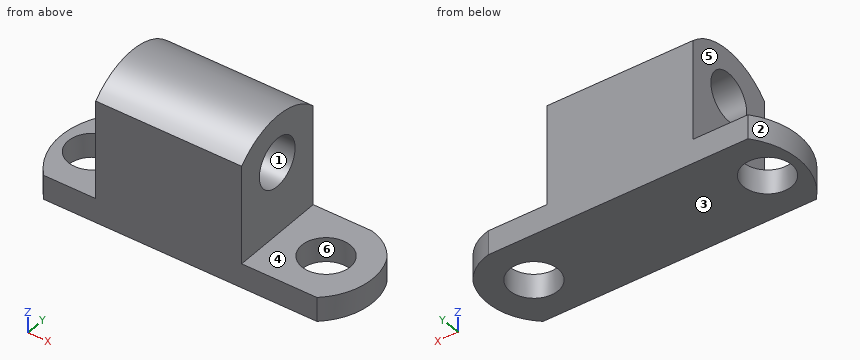
from build123d import *

# Parameters (mm, degrees)
F0_W      = 82.55
F0_H      = 38.1
F1_DEPTH  = 25.4
F2_W      = 25.4
F2_H      = 31.75
F3_DEPTH  = 25.4
F4_W      = 19.05
F4_H      = 31.75
F5_DEPTH  = 25.4
F6_R      = 6.35
F7_DEPTH  = 25.4
F8_R      = 6.35
F9_DEPTH  = 25.4
F11_DEPTH = 38.1
F12_R     = 6.35
F13_DEPTH = 50.8
F15_DEPTH = 50.8
F17_DEPTH = 50.8
F19_DEPTH = 25.4


with BuildPart() as f1:
    # F0 (on Front) → F1 (new body)
    with BuildSketch(Plane.XZ):
        with Locations((41.275, 19.05)):
            Rectangle(F0_W, F0_H)
    extrude(amount=F1_DEPTH)

    # F2 (on face) → F3 (cut)
    with BuildSketch(Plane.XZ.offset(25.4)):
        with Locations((69.85, 22.225)):
            Rectangle(F2_W, F2_H)
    extrude(amount=-F3_DEPTH, mode=Mode.SUBTRACT)

    # F4 (on face) → F5 (cut)
    with BuildSketch(Plane.XZ.offset(25.4)):
        with Locations((9.525, 22.225)):
            Rectangle(F4_W, F4_H)
    extrude(amount=-F5_DEPTH, mode=Mode.SUBTRACT)

    # F6 (on face) → F7 (cut)
    with BuildSketch(Plane.XY.offset(6.35)):
        with Locations((69.85, -12.7)):
            Circle(F6_R)
    extrude(amount=-F7_DEPTH, mode=Mode.SUBTRACT)

    # F8 (on face) → F9 (cut)
    with BuildSketch(Plane.XY.offset(6.35)):
        with Locations((8.8900124169, -12.7158843127)):
            Circle(F8_R)
    extrude(amount=-F9_DEPTH, mode=Mode.SUBTRACT)

    # F10 (on face) → F11 (cut)
    with BuildSketch(Plane(origin=(19.05, 0, 0), x_dir=(0, -1, 0), z_dir=(-1, 0, 0))):
        with BuildLine():
            ThreePointArc((0, 32.5376726687), (12.769661319, 37.7082569413), (25.4, 32.2060994804))
            Line((25.4, 32.2060994804), (25.4, 38.1))
            Line((25.4, 38.1), (0, 38.1))
            Line((0, 38.1), (0, 32.5376726687))
        make_face()
    extrude(amount=-F11_DEPTH, mode=Mode.SUBTRACT)

    # F12 (on face) → F13 (cut)
    with BuildSketch(Plane.YZ.offset(57.15)):
        with Locations((-12.769661319, 25.3998726321)):
            Circle(F12_R)
    extrude(amount=-F13_DEPTH, mode=Mode.SUBTRACT)

    # F14 (on face) → F15 (cut)
    with BuildSketch(Plane.XY.offset(6.35)):
        with BuildLine():
            ThreePointArc((5.4768570699, -25.4), (0.241233284, -12.8565406161), (4.6525248326, 0))
            Line((4.6525248326, 0), (0, 0))
            Line((0, 0), (0, -25.4))
            Line((0, -25.4), (5.4768570699, -25.4))
        make_face()
    extrude(amount=-F15_DEPTH, mode=Mode.SUBTRACT)

    # F16 (on face) → F17 (cut)
    with BuildSketch(Plane.XY.offset(6.35)):
        with BuildLine():
            ThreePointArc((75.7511779666, 0), (82.4170329692, -12.4504834206), (76.7815932631, -25.4))
            Line((76.7815932631, -25.4), (82.55, -25.4))
            Line((82.55, -25.4), (82.55, 0))
            Line((82.55, 0), (75.7511779666, 0))
        make_face()
    extrude(amount=-F17_DEPTH, mode=Mode.SUBTRACT)

    # F18 (on face) → F19 (cut)
    with BuildSketch(Plane.XY.offset(6.35)):
        with BuildLine():
            ThreePointArc((72.4261626601, 0), (77.2939859852, -2.2026454539), (80.8707558382, -6.1717849498))
            ThreePointArc((80.8707558382, -6.1717849498), (78.6988634902, -2.7641270855), (75.7511779666, 0))
            Line((75.7511779666, 0), (72.4261626601, 0))
        make_face()
    extrude(amount=-F19_DEPTH, mode=Mode.SUBTRACT)


solid = f1.part
The listing builds one solid part. Answer for the finished solid, in the listing's coordinates (mm). Face numbers are marked on the shaded views. A direction names the side the tool comes from. Coordinates: 2 decimals unless noted, no trailing zeros. Loops run counter-clockwise (first coordinate to the right, second up) from the corner with the lowest first, then second, coordinate; pieces in that order, holes last. Notation, with made-up numbers: (85, 77.25) -> (127, 77.25) arc R20 ccw to (127, 114.25) -> close; hole circle Ø10 at (-37, -14). An arc over 180 degrees is marked (long way). Answer in a Markdown table with one row per item. Add a question column.
1. The part is cut by section B-B, the plane z = 23. Write down the section's boundary in (x, y).
2. Flat-ended cylindrical pins translate along their axes: P1, Ø7.5, axis at y = -10.5, z = 19, coming from the -X side; P2, Ø12.5, axis at y = -8.5, z = 16.5, coming from the +X side; P3, Ø1.5, axis at x = 32.5, y = -3.5, coming from the +Z side. Find the tip coordinate at first contact, or state that the pin passes through.
3. The part is cut by section D-D, the plane x = 33.5. Write down the section's boundary in (y, z), then the cut area to 3 significant figures.
4. Consider line 1 (Y direction, x = 69.85, z = 4); line 2 (X direction, y = -15.5, z = 35); line 3 (Z direction, x = 50, y = -13). Determine where each line is inside the solid, lowest interval first. Write a range as [from, to].
5. The part is cut by section A-A, the plane x = 69.85. Write down the section's boundary in (y, z), then the cut area to 3 significant figures.
6. Determine the mould class of the marked faces 1, 2 and 3 for opening direction Y: +Y half, -Y half, draft (parallel to the pull), parting line (faces both ways), or undercut.
7. For the marked faces 4, 5 and 6, determine the directions among +Z, -Z, +X, -X, +Y, -Y from which every point of the face is accessible in a straight line to the end or side of a thin tool.
8. The part is cut by section C-C, the plane y = -3.25. Write down the section's boundary in (x, z).
Answer below:
| question | item | result |
|---|---|---|
| 1 | outline | (19.05, -25.4) -> (57.15, -25.4) -> (57.15, -18.65) -> (19.05, -18.65) -> close; (19.05, -6.89) -> (57.15, -6.89) -> (57.15, 0) -> (19.05, 0) -> close |
| 2 | P1 | x = 19.05 |
| 2 | P2 | x = 57.15 |
| 2 | P3 | z = 35.66 |
| 3 | outline | (-25.4, 0) -> (0, 0) -> (0, 32.54) arc R17.78 ccw to (-25.4, 32.21) -> close; hole circle Ø12.7 at (-12.77, 25.4) |
| 3 | area | 789 mm2 |
| 4 | line 1 | [-25.4, -19.05], [-6.35, 0] |
| 4 | line 2 | [19.05, 57.15] |
| 4 | line 3 | [0, 19.05], [31.75, 37.7] |
| 5 | outline | (-25.4, 0) -> (-19.05, 0) -> (-19.05, 6.35) -> (-25.4, 6.35) -> close; (-6.35, 0) -> (0, 0) -> (0, 6.35) -> (-6.35, 6.35) -> close |
| 5 | area | 80.6 mm2 |
| 6 | face 1 | undercut |
| 6 | face 2 | parting line |
| 6 | face 3 | draft |
| 7 | face 4 | +Z, +X, +Y, -Y |
| 7 | face 5 | +Z, -X, +Y, -Y |
| 7 | face 6 | +Z, -Z |
| 8 | outline | (2.47, 0) -> (78.55, 0) -> (78.55, 6.35) -> (57.15, 6.35) -> (57.15, 35.09) -> (19.05, 35.09) -> (19.05, 6.35) -> (2.47, 6.35) -> close |
